Model file for the job. Use its own axes, mm. Face numbers are marked on the shaded views. Round coordinates to 2 decimals unless told otherwise and drop trailing zeros. Order: outer loops, then holes, each group sorted by start corner. A loop starts at its lowest first (then second) coordinate and runs counter-clockwise, first axis right, second up. Notation, with made-up numbers: (-35, 0.25) - (-7, 0.25) arc R16 cw to (-7, 30.25) - close; hole circle Ø8 at (-1.75, -5). An arc over 180 degrees is marked (long way). Use one line per item in the form item = value.
Autodesk Inventor part; units mm, degrees
ref_plane "YZ Plane" through (0, 0, 0) normal (1, 0, 0) x (0, 1, 0)
ref_plane "XZ Plane" through (0, 0, 0) normal (0, 1, 0) x (-1, 0, 0)
ref_plane "XY Plane" through (0, 0, 0) normal (0, 0, 1) x (1, 0, 0)
sketch "Sketch1" plane through (0, 0, 0) normal (0, 0, 1) x (1, 0, 0)
  line L0 (-10, 0) -> (-7.8787, 2.1213)
  line L1 (-7.8787, 2.1213) -> (-107.8787, 102.1213)
  line L2 (-107.8787, 102.1213) -> (-110, 100)
  line L3 (-110, 100) -> (-10, 0)
  line L4 (-10, 0) -> (0, 0) construction
  dimension "d24" = 10
  dimension "d25" = 3
  dimension "d26" = 45
  dimension "d27" = 100
extrude "Extrusion1" add sketch "Sketch1" along normal mid plane 100
chamfer "Chamfer1" distance 10 angle 45 4 edges at (-108.9393, 101.0607, 50) (-8.9393, 1.0607, 50) (-8.9393, 1.0607, -50) (-108.9393, 101.0607, -50)
sketch "Sketch2" plane through (0, 0, 0) normal (1, 0, 0) x (0, 1, 0)
  arc A0 (51.5, -1.3229) -> (51.5, 1.3229) centre (50, 0) ccw
  line L0 (55, -2.0711) -> (52.0711, -5)
  line L1 (52.0711, -5) -> (47.9289, -5)
  line L2 (47.9289, -5) -> (45, -2.0711)
  line L3 (45, -2.0711) -> (45, 2.0711)
  line L4 (45, 2.0711) -> (47.9289, 5)
  line L5 (47.9289, 5) -> (52.0711, 5)
  line L6 (52.0711, 5) -> (55, 2.0711)
  line L7 (55, 2.0711) -> (55, -2.0711)
  line L8 (51.5, 1.3229) -> (51.5, -1.3229)
  line L9 (48.5, 1.3229) -> (48.5, -1.3229)
  arc A1 (48.5, -1.3229) -> (51.5, -1.3229) centre (50, 0) ccw
  arc A2 (51.5, 1.3229) -> (48.5, -1.3229) centre (50, 0) ccw
  circle A3 centre (85, 30) radius 4
  circle A4 centre (85, -30) radius 4
  circle A5 centre (22, 30) radius 4
  circle A6 centre (22, -30) radius 4
  line L10 (10, 40) -> (90, 40)
  line L11 (90, 40) -> (90, -40)
  line L12 (90, -40) -> (10, -40)
  line L13 (10, -40) -> (10, 40)
  line L14 (10, 40) -> (90, -40) construction
  line L15 (90, 40) -> (10, -40) construction
  circle A7 centre (50, 40) radius 20
  circle A8 centre (50, -40) radius 20
  circle A9 centre (90, 0) radius 20
  circle A10 centre (50, 0) radius 4.61
  circle A11 centre (10, 0) radius 20
  point P0 (0, 0)
  point P1 (0, 0)
  point P2 (50, 0)
  dimension "d8" = 50
  dimension "d10" = 4
  dimension "d11" = 5
  dimension "d14" = 3
  dimension "d15" = 30
  dimension "d16" = 30
  dimension "d17" = 35
  dimension "d18" = 28
  dimension "d19" = 8
  dimension "d28" = 80
  dimension "d29" = 80
  dimension "d35" = 9.22
  dimension "d38" = 40
extrude "Extrusion2" add sketch "Sketch2" against normal up to next contours L8 A0 | A1 L9 A2 L8 | A2 L9 | L0 L1 L2 L3 L4 L5 L6 L7 | A10
extrude "Extrusion3" add sketch "Sketch2" against normal blind 3 contours A7 L10 | L10 L11 A9 L12 A8 L13 A11 A7 | L11 A9 | A11 L13 | L12 A8 picked at (44.8162, 33.9837) picked at (86.9018, -5.903) picked at (22.2846, 1.4835) picked at (43.3333, -31.1584)
extrude "Extrusion4" add sketch "Sketch2" against normal up to next contours A3 | A4 | A5 | A6
extrude "Extrusion5" cut sketch "Sketch2" against normal up to surface (3 mm away) contours A7 L10 | L10 A7 | A9 L11 | L11 A9 | A11 L13 | L13 A11 | A8 L12 | L12 A8
fillet "Fillet2" radius 8 12 edges at (-1.5, 30, 40) (-1.5, 70, 40) (-1.5, 10, 40) (-1.5, 10, -40) (-1.5, 70, -40) (-1.5, 30, -40) (-1.5, 90, -40) (-1.5, 90, 20) (-1.5, 90, -20) (-1.5, 90, 40) (-1.5, 10, 20) (-1.5, 10, -20)
extrude "Extrusion7" add sketch "Sketch2" along normal blind 10 contours L0 L1 L2 L3 L4 L5 L6 L7
extrude "Extrusion8" add sketch "Sketch2" along normal blind 8.25 contours A10
extrude "Extrusion9" add sketch "Sketch2" along normal blind 6.22 contours L8 A0 | A2 L9
properties part number "MIRROR MOUNT"
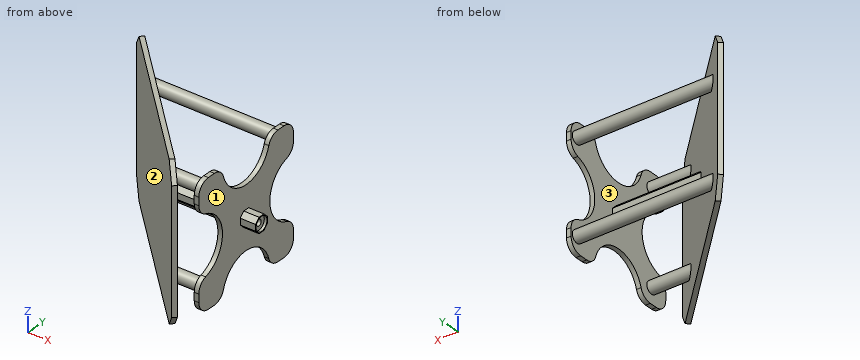
(1) Pin check, flat tips, straight feed: pin 1 (4.5 mm diameter, centred on y = 50, z = 0, fed in from +X); pin 2 (3.5 mm diameter, centred on x = 5, y = 50, fed in from -Z); pin 3 (2 mm diameter, centred on x = -21.5, y = 50.5, fed in from +Z); pin 4 (6 mm diameter, centred on x = -46, y = 29, fed in from -Z). Stop position of each tip, or through.
Report:
pin_1 = 8.25
pin_2 = -5
pin_3 = 5
pin_4 = through
(2) Slice it at B-B on y = 67. Give the cut face in (x, z), then the cut area to 3 significant figures.
Report:
outline = (-77, -50) - (-72.76, -50) - (-72.76, 50) - (-77, 50) - close; (-3, -29.46) - (0, -29.46) - (0, 29.46) - (-3, 29.46) - close
area = 601 mm2
(3) Probe probe 1 along Y at (x, z) = (2.25, 0); probe 2 along Z at (x, y) = (3, 50); probe 3 along Y at (x, z) = (6.25, 0). List the from-to ranges inside material, lowest first. Write a range as [from, to].
Report:
probe_1 = [45, 48.5], [51.5, 55]
probe_2 = [-5, -2], [2, 5]
probe_3 = [45, 48], [52, 55]
(4) Pull direction X, two halves, no side cores. Call the marked faces 1, 2 and 3: released by +X, released by -X, zero draft, split by the parting line, or undercut.
Report:
face_1 = released by +X
face_2 = released by -X
face_3 = undercut
(5) Slice it at D-D on z = 23.5. Give the cut face in (x, y).
Report:
outline = (-110, 100) - (-10, 0) - (-7.88, 2.12) - (-107.88, 102.12) - close; (-3, 10.73) - (0, 10.73) - (0, 38.7) - (-3, 38.7) - close; (-3, 61.3) - (0, 61.3) - (0, 89.27) - (-3, 89.27) - close
(6) Slice it at C-C on x = -70. Give the cut face in (y, z), then the cut area to 3 significant figures.
Report:
outline = (60, -50) - (64.24, -50) - (64.24, 50) - (60, 50) - close; circle Ø8 at (85, -30); circle Ø8 at (85, 30)
area = 525 mm2
(7) Slice it at A-A on x = -29.5. Give the cut face in (y, z), then the cut area to 3 significant figures.
Report:
outline = (19.5, -50) - (23.74, -50) - (23.74, -33.6) arc R4 ccw to (23.74, -26.4) - (23.74, 26.4) arc R4 ccw to (23.74, 33.6) - (23.74, 50) - (19.5, 50) - close; (45, -2.07) - (47.93, -5) - (52.07, -5) - (55, -2.07) - (55, 2.07) - (52.07, 5) - (47.93, 5) - (45, 2.07) - close; circle Ø8 at (85, -30); circle Ø8 at (85, 30)
area = 631 mm2
